from build123d import *

# Parameters (mm, degrees)
SKETCH11_W                    = 150.473018286
SKETCH11_H                    = 83.2350749
BOSS_EXTRUDE1_DEPTH           = 10
SKETCH13_W                    = 15
SKETCH13_H                    = 83.2350749
BOSS_EXTRUDE2_DEPTH           = 20
BOSS_EXTRUDE2_DRAFT           = 10
BOSS_EXTRUDE2_PROFILE_2_DEPTH = 20
BOSS_EXTRUDE2_PROFILE_2_DRAFT = 10
SKETCH16_R                    = 10.695894528
SKETCH16_W                    = 49.642014298
SKETCH16_H                    = 21.391789056
CUT_EXTRUDE17_DEPTH           = 10


with BuildPart() as part:
    # Sketch11 → Boss-Extrude1 (new body)
    with BuildSketch(Plane(origin=(0, 0, 0), x_dir=(1, 0, 0), z_dir=(0, 1, 0))):
        Rectangle(SKETCH11_W, SKETCH11_H)
    extrude(amount=BOSS_EXTRUDE1_DEPTH)


with BuildPart() as boss_extrude2_tool:
    # Sketch13 → Boss-Extrude2 (with draft: the straight prism first)
    with BuildSketch(Plane(origin=(0, 10, 0), x_dir=(1, 0, 0), z_dir=(0, 1, 0))):
        with Locations((-67.736509143, 0)):
            Rectangle(SKETCH13_W, SKETCH13_H)
    extrude(amount=BOSS_EXTRUDE2_DEPTH)
    # Boss-Extrude2: the draft: its side faces are tilted about the plane it starts from
    boss_extrude2_sides = [boss_extrude2_tool.faces().sort_by_distance(p)[0] for p in [
        (-75.236509143, 20, 0),
        (-67.736509143, 20, 41.61753745),
        (-60.236509143, 20, 0),
        (-67.736509143, 20, -41.61753745),
    ]]
    draft(boss_extrude2_sides, Plane(origin=(0, 10, 0), x_dir=(1, 0, 0), z_dir=(0, 1, 0)), BOSS_EXTRUDE2_DRAFT)


with BuildPart() as part_1:
    add(part.part)

    # Boss-Extrude2: add boss_extrude2_tool
    add(boss_extrude2_tool.part)


with BuildPart() as boss_extrude2_profile_2_tool:
    # Sketch13 → Boss-Extrude2 profile 2 (with draft: the straight prism first)
    with BuildSketch(Plane(origin=(0, 10, 0), x_dir=(1, 0, 0), z_dir=(0, 1, 0))):
        with Locations((67.736509143, 0)):
            Rectangle(SKETCH13_W, SKETCH13_H)
    extrude(amount=BOSS_EXTRUDE2_PROFILE_2_DEPTH)
    # Boss-Extrude2 profile 2: the draft: its side faces are tilted about the plane it starts from
    boss_extrude2_profile_2_sides = [boss_extrude2_profile_2_tool.faces().sort_by_distance(p)[0] for p in [
        (67.736509143, 20, -41.61753745),
        (60.236509143, 20, 0),
        (67.736509143, 20, 41.61753745),
        (75.236509143, 20, 0),
    ]]
    draft(boss_extrude2_profile_2_sides, Plane(origin=(0, 10, 0), x_dir=(1, 0, 0), z_dir=(0, 1, 0)), BOSS_EXTRUDE2_PROFILE_2_DRAFT)


with BuildPart() as part_2:
    add(part_1.part)

    # Boss-Extrude2 profile 2: add boss_extrude2_profile_2_tool
    add(boss_extrude2_profile_2_tool.part)

    # Sketch16 → Cut-Extrude17 (cut)
    with BuildSketch(Plane(origin=(0, 10, 0), x_dir=(1, 0, 0), z_dir=(0, 1, 0))):
        with Locations((24.821007149, 0)):
            Circle(SKETCH16_R)
        with Locations((-24.821007149, 0)):
            Circle(SKETCH16_R)
        Rectangle(SKETCH16_W, SKETCH16_H)
    extrude(amount=-CUT_EXTRUDE17_DEPTH, mode=Mode.SUBTRACT)


solid = part_2.part
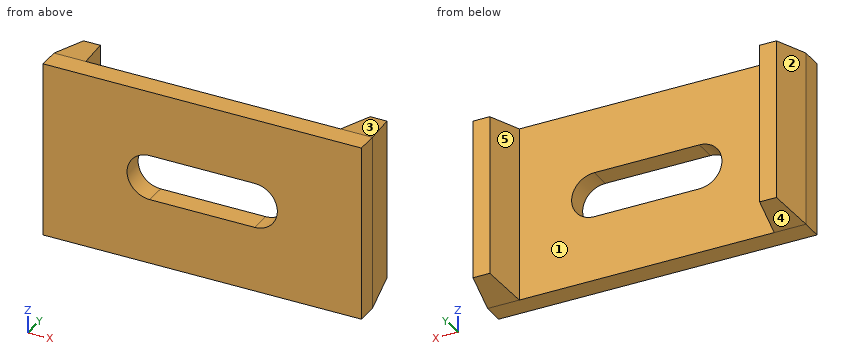
The listing builds one solid part. Answer for the finished solid, in the listing's coordinates (mm). Face numbers are marked on the shaded views. A direction names the side the tool comes from. Coordinates: 2 decimals unless noted, no trailing zeros. Loops run counter-clockwise (first coordinate to the right, second up) from the corner with the lowest first, then second, coordinate; pieces in that order, holes last. Notation, with made-up numbers: (8.25, 71.25) -> (23.25, 71.25) arc R20 cw to (23.25, 93.25) -> close; hole circle Ø8 at (50, -32.5). An arc over 180 degrees is marked (long way). Answer in a Markdown table with one row per item. Add a question column.
1. The part is cut by section C-C, the plane y = 3.25. Write down the section's boundary in (x, z), then the cut area to 3 significant figures.
2. A flat-ended cylindrical pin translates along its axis: P1, Ø12, axis at y = 13.5, z = 1, coming from the +X side. Find the tip coordinate at first contact, or state that the pin passes through.
3. For the marked faces 4 and 5, determine the directions among +Z, -Z, +X, -X, +Y, -Y from which every point of the face is accessible in a straight line to the end or side of a thin tool.
4. The part is cut by section B-B, the plane x = 17. Write down the section's boundary in (y, z), then the cut area to 3 significant figures.
5. Determine the mould class of the marked faces 1, 2 and 3 for opening direction X: +X half, -X half, draft (parallel to the pull), parting line (faces both ways), or undercut.
6. The part is cut by section D-D, the plane y = 23. Write down the section's boundary in (x, z).
7. Consider line 1 (Z direction, x = -22.5, y = 5.5); line 2 (Y direction, x = -53.5, z = -29.5); line 3 (X direction, y = 18, z = -5.5). Determine where each line is inside the solid, lowest interval first. Write a range as [from, to].
8. The part is cut by section A-A, the plane z = 0. Write down the section's boundary in (x, y).
Answer below:
| question | item | result |
|---|---|---|
| 1 | outline | (-75.24, -41.62) -> (75.24, -41.62) -> (75.24, 41.62) -> (-75.24, 41.62) -> close; hole (-24.82, -10.7) -> (24.82, -10.7) arc R10.7 ccw to (24.82, 10.7) -> (-24.82, 10.7) arc R10.7 ccw to start |
| 1 | area | 11,100 mm2 |
| 2 | P1 | x = 75.24 |
| 3 | face 4 | -Z, +X, -X, +Y |
| 3 | face 5 | +Z, -Z, +Y |
| 4 | outline | (0, -41.62) -> (10, -41.62) -> (10, -10.7) -> (0, -10.7) -> close; (0, 10.7) -> (10, 10.7) -> (10, 41.62) -> (0, 41.62) -> close |
| 4 | area | 618 mm2 |
| 5 | face 1 | undercut |
| 5 | face 2 | -X half |
| 5 | face 3 | draft |
| 6 | outline | (-72.94, -39.33) -> (-62.53, -39.33) -> (-62.53, 39.33) -> (-72.94, 39.33) -> close; (62.53, -39.33) -> (72.94, -39.33) -> (72.94, 39.33) -> (62.53, 39.33) -> close |
| 7 | line 1 | [-41.62, -10.7], [10.7, 41.62] |
| 7 | line 2 | [0, 10] |
| 7 | line 3 | [-73.83, -61.65], [61.65, 73.83] |
| 8 | outline | (-75.24, 0) -> (-35.52, 0) -> (-35.52, 10) -> (-60.24, 10) -> (-63.76, 30) -> (-71.71, 30) -> (-75.24, 10) -> close; (35.52, 0) -> (75.24, 0) -> (75.24, 10) -> (71.71, 30) -> (63.76, 30) -> (60.24, 10) -> (35.52, 10) -> close |
